Could you check a few things on this model? Use its own coordinates, in mm. Coordinates: 2 decimals unless noted, no trailing zeros. Write each loop counter-clockwise with the first axis right and the second up, starting at its lowest first coordinate (ties: lowest second). Pieces come first, ordered by that corner, then holes. Notation, with made-up numbers: M 53,74.25 L 109,74.25 A19 ccw 109,96.25 Z; hole C 87.5,10 d2. An arc over 180 degrees is marked long. Answer as CSV lines item,"result". Start each with the question number.
Item 1: Suppose I cut it at B-B, the plane x = 0. Write out the boundary of the cut face in (y, z).
Item 2: Suppose I cut it at C-C, the plane x = -62.5. Write out the boundary of the cut face in (y, z), and give its area (3 significant figures).
Item 3: Suppose I cut it at A-A, the plane y = -15. Write out the boundary of the cut face in (x, z).
Item 4: Suppose I cut it at D-D, the plane x = 90. Write out the boundary of the cut face in (y, z).
Item 5: If I drill on line 1 along X through (y, z) = (29.5, 5); line 2 along Y through (x, z) = (10, 5.5); line 3 along Y through (x, z) = (77.5, 1), over which ranges is the centre line in solid material (lowest first)? Write a range as [from, to].
Item 6: We'd pull the mould along X, two halves only. Please class faces 1 (the flat face through (88, 31, 2)), 2 (the cylindrical face through (-94.49, -37.15, 2.96)), 3 (the cylindrical face through (94.496, -29.698, 3.014)), 4 (the flat face through (-95, 2.5, 0)): +X half, -X half, draft (parallel to the pull), parting line (faces both ways), or undercut.
Item 7: I'm going to push a flat-ended pin straight in: P1, Ø4.5, axis at x = -79, y = -31, coming from the -Z side. Where does the tip first touch, or does it pass through?
Autodesk Inventor part; units mm, degrees
ref_plane "YZ Plane" through (0, 0, 0) normal (1, 0, 0) x (0, 1, 0)
ref_plane "XZ Plane" through (0, 0, 0) normal (0, 1, 0) x (-1, 0, 0)
ref_plane "XY Plane" through (0, 0, 0) normal (0, 0, 1) x (1, 0, 0)
ref_plane "Work Plane1" through (0, 0, 0) normal (0, 0, 1) x (1, 0, 0)
sketch "Sketch1" plane through (0, 0, 0) normal (0, 0, 1) x (1, 0, 0)
  arc A0 (87.5, -38) -> (95.5, -30) centre (87.5, -30) ccw
  line L0 (87.5, -38) -> (-87.5, -38)
  arc A1 (-95.5, -30) -> (-87.5, -38) centre (-87.5, -30) ccw
  line L1 (-95.5, -30) -> (-95.5, 30)
  arc A2 (-87.5, 38) -> (-95.5, 30) centre (-87.5, 30) ccw
  line L2 (-87.5, 38) -> (87.5, 38)
  arc A3 (95.5, 30) -> (87.5, 38) centre (87.5, 30) ccw
  line L3 (95.5, 30) -> (95.5, -30)
  line L4 (-87.5, -40) -> (87.5, -40)
  arc A4 (87.5, -40) -> (97.5, -30) centre (87.5, -30) ccw
  line L5 (97.5, -30) -> (97.5, 30)
  arc A5 (97.5, 30) -> (87.5, 40) centre (87.5, 30) ccw
  line L6 (87.5, 40) -> (-87.5, 40)
  arc A6 (-87.5, 40) -> (-97.5, 30) centre (-87.5, 30) ccw
  line L7 (-97.5, 30) -> (-97.5, -30)
  arc A7 (-97.5, -30) -> (-87.5, -40) centre (-87.5, -30) ccw
  point P0 (0, 0)
extrude "Extrusion1" add sketch "Sketch1" along normal blind 4
sketch "Sketch2" plane through (0, 0, 4) normal (0, 0, 1) x (1, 0, 0)
  arc A0 (87.5, -40) -> (97.5, -30) centre (87.5, -30) ccw
  line L0 (97.5, -30) -> (97.5, 30)
  arc A1 (97.5, 30) -> (87.5, 40) centre (87.5, 30) ccw
  line L1 (87.5, 40) -> (-87.5, 40)
  arc A2 (-87.5, 40) -> (-97.5, 30) centre (-87.5, 30) ccw
  line L2 (-97.5, 30) -> (-97.5, -30)
  arc A3 (-97.5, -30) -> (-87.5, -40) centre (-87.5, -30) ccw
  line L3 (-87.5, -40) -> (87.5, -40)
  line L4 (-95.5, -30) -> (-95.5, 30)
  arc A4 (-87.5, 38) -> (-95.5, 30) centre (-87.5, 30) ccw
  line L5 (-87.5, 38) -> (87.5, 38)
  arc A5 (95.5, 30) -> (87.5, 38) centre (87.5, 30) ccw
  line L6 (95.5, 30) -> (95.5, -30)
  arc A6 (87.5, -38) -> (95.5, -30) centre (87.5, -30) ccw
  line L7 (87.5, -38) -> (-87.5, -38)
  arc A7 (-95.5, -30) -> (-87.5, -38) centre (-87.5, -30) ccw
  circle A8 centre (-80, -29.5) radius 2.15
  circle A9 centre (0, -29.5) radius 2.15
  circle A10 centre (-80, 29.5) radius 2.15
  circle A11 centre (0, 29.5) radius 2.15
  circle A12 centre (10, 29.5) radius 2.15
  circle A13 centre (10, -29.5) radius 2.15
  circle A14 centre (90, -29.5) radius 2.15
  circle A15 centre (90, 29.5) radius 2.15
  circle A16 centre (-80, 29.5) radius 1.75
  circle A17 centre (-80, -29.5) radius 1.75
  circle A18 centre (0, -29.5) radius 1.75
  circle A19 centre (10, -29.5) radius 1.75
  circle A20 centre (0, 29.5) radius 1.75
  circle A21 centre (10, 29.5) radius 1.75
  circle A22 centre (90, 29.5) radius 1.75
  circle A23 centre (90, -29.5) radius 1.75
  point P0 (0, 0)
  dimension "d2" = 3.5
  dimension "d3" = 3.5
  dimension "d4" = 3.5
  dimension "d5" = 3.5
  dimension "d6" = 3.5
  dimension "d7" = 3.5
  dimension "d8" = 3.5
  dimension "d9" = 3.5
extrude "Extrusion2" add sketch "Sketch2" along normal blind 2 contours L3 A3 L2 A2 L1 A1 L0 A0 | L4 A4 L5 A5 L6 A6 L7 A7
sketch "Sketch3" plane through (0, 0, 4) normal (0, 0, -1) x (-1, 0, 0)
  circle A0 centre (80, 29.5) radius 2.15
  circle A1 centre (80, 29.5) radius 4.5
  circle A2 centre (80, -29.5) radius 2.15
  circle A3 centre (80, -29.5) radius 4.5
  circle A4 centre (0, 29.5) radius 2.15
  circle A5 centre (0, 29.5) radius 4.5
  circle A6 centre (0, -29.5) radius 2.15
  circle A7 centre (0, -29.5) radius 4.5
  circle A8 centre (-10, 29.5) radius 2.15
  circle A9 centre (-10, 29.5) radius 4.5
  circle A10 centre (-10, -29.5) radius 2.15
  circle A11 centre (-10, -29.5) radius 4.5
  circle A12 centre (-90, 29.5) radius 2.15
  circle A13 centre (-90, 29.5) radius 4.5
  circle A14 centre (-90, -29.5) radius 2.15
  circle A15 centre (-90, -29.5) radius 4.5
  point P0 (0, 0)
  dimension "d17" = 9
extrude "Extrusion3" add sketch "Sketch3" along normal blind 2
sketch "Sketch4" plane through (0, 0, 4) normal (0, 0, -1) x (-1, 0, 0)
  line L0 (75, 36) -> (-75, 36)
  line L1 (-75, 36) -> (-75, 38)
  line L2 (-75, 38) -> (75, 38)
  line L3 (75, 38) -> (75, 36)
  line L4 (87.5, 38) -> (-87.5, 38)
  line L5 (-75, -36) -> (75, -36)
  line L6 (75, -38) -> (-75, -38)
  line L7 (75, -36) -> (75, -38)
  line L8 (-75, -38) -> (-75, -36)
  line L9 (-95.5, 20) -> (-93.5, 20)
  line L10 (-93.5, 20) -> (-93.5, -20)
  line L11 (-93.5, -20) -> (-95.5, -20)
  line L12 (-95.5, -20) -> (-95.5, 20)
  line L13 (-95.5, 30) -> (-95.5, -30)
  line L14 (93.5, 20) -> (95.5, 20)
  line L15 (95.5, 20) -> (95.5, -20)
  line L16 (95.5, -20) -> (93.5, -20)
  line L17 (93.5, -20) -> (93.5, 20)
  line L18 (95.5, -30) -> (95.5, 30)
  point P0 (0, 0)
  point P1 (0, 38)
  point P2 (0, -38)
  point P3 (-95.5, 0)
  point P4 (95.5, 0)
  dimension "d22" = 2
  dimension "d23" = 150
  dimension "d26" = 360
  dimension "d30" = 2
  dimension "d31" = 40
extrude "Extrusion4" add sketch "Sketch4" along normal blind 6 contours L0 L1 L2 L3 | L5 L7 L6 L8 | L14 L15 L16 L17
sketch "Sketch7" plane through (0, 0, -2) normal (0, 0, -1) x (-1, 0, 0)
  line L0 (93.5, -20) -> (93.5, 20)
  line L1 (97.5, 30) -> (97.5, -30)
  line L2 (93.5, 2.5) -> (97.5, 2.5)
  line L3 (97.5, 2.5) -> (97.5, -2.5)
  line L4 (97.5, -2.5) -> (93.5, -2.5)
  line L5 (93.5, -2.5) -> (93.5, 2.5)
  point P0 (0, 0)
  point P1 (93.5, 0)
  dimension "d38" = 5
extrude "Extrusion7" cut sketch "Sketch7" against normal blind 4
properties part number "led 7 seg v3_bottom"
Ans:
1,outline,"M -40,0 L -38,0 L -38,-2 L -36,-2 L -36,4 L -34,4 L -34,2 L -31.65,2 L -31.65,6 L -40,6 Z; M -27.35,2 L -25,2 L -25,4 L 25,4 L 25,2 L 27.35,2 L 27.35,6 L -27.35,6 Z; M 31.65,2 L 34,2 L 34,4 L 36,4 L 36,-2 L 38,-2 L 38,0 L 40,0 L 40,6 L 31.65,6 Z"
2,outline,"M -40,0 L -38,0 L -38,-2 L -36,-2 L -36,4 L 36,4 L 36,-2 L 38,-2 L 38,0 L 40,0 L 40,6 L -40,6 Z"
2,area,"200 mm^2"
3,outline,"M -97.5,0 L -95.5,0 L -95.5,-2 L -93.5,-2 L -93.5,4 L 95.5,4 L 95.5,0 L 97.5,0 L 97.5,6 L -97.5,6 Z"
4,outline,"M -39.68,0 L -37.6,0 L -37.6,4 L -34,4 L -34,2 L -31.65,2 L -31.65,6 L -39.68,6 Z; M -27.35,2 L -25,2 L -25,4 L 25,4 L 25,2 L 27.35,2 L 27.35,6 L -27.35,6 Z; M 31.65,2 L 34,2 L 34,4 L 37.6,4 L 37.6,0 L 39.68,0 L 39.68,6 L 31.65,6 Z"
5,line 1,"x = [-97.5, -82.15], [-77.85, -2.15], [2.15, 7.85], [12.15, 87.85], [92.15, 97.5]"
5,line 2,"y = [-40, -31.65], [-27.35, 27.35], [31.65, 40]"
5,line 3,"y = [-40, -38], [38, 40]"
6,face 1,"undercut"
6,face 2,"-X half"
6,face 3,"undercut"
6,face 4,"draft"
7,P1,"stops at z = 2"
